Part model, mm, in its own coordinate system. Face numbers are marked on the shaded views. A direction names the side the tool comes from. Coordinates: 2 decimals unless noted, no trailing zeros. Write each loop counter-clockwise with the first axis right and the second up, starting at its lowest first coordinate (ties: lowest second). Pieces come first, ordered by that corner, then holes. Notation, with made-up numbers: M 81.5,67.25 L 92.5,67.25 A10 ccw 92.5,73.25 Z; hole C 82.25,-39 d4. An arc over 180 degrees is marked long. Use a Markdown table: item, result. Add a question column.
Q1. Mould opens along X. For the marked faces 3, 4, 5 and 6 say: released by +X, released by -X, zero draft, split by the parting line, or undercut.
Q2. Pin check, flat tip, straight feed: pin 1 Ø5.5 at (y, z) = (26, 93.5) entering from +X. Stop position of the tip, or through.
Q3. Slice it at A-A on x = 350. Write the cut outline in (y, z), then the cut area to 3 significant figures.
Q4. Tool access for the marked faces 1 and 2: list every direction of +Z, -Z, +X, -X, +Y, -Y with a clear straight run to the whole face (end or side of a thin tool).
Q5. Wall check: L1, parallel to Y at x = 385, z = -39.5; L2, parallel to Z at x = 312, y = 110; L3, parallel to Z at x = 404, y = 32. Give the ranges that are in metal, low to high. Write a range as from..to.
Q6. Slice it at B-B on y = 112.5. Count the separate pieces of the cut face and the enclosed holes in it, then the cut area to 3 significant figures.
from build123d import *

# Parameters (mm, degrees)
SKETCH_1_W      = 740
SKETCH_1_H      = 190
EXTRUDE_1_DEPTH = 100
SKETCH_2_R      = 14.812408038
EXTRUDE_2_DEPTH = 20
SKETCH_3_W      = 180
SKETCH_3_H      = 100
EXTRUDE_3_DEPTH = 100


with BuildPart() as part:
    # 草图1 → 凸台-拉伸1 (new body)
    with BuildSketch(Plane(origin=(0, 0, 0), x_dir=(1, 0, 0), z_dir=(0, 1, 0))):
        Rectangle(SKETCH_1_W, SKETCH_1_H)
    extrude(amount=EXTRUDE_1_DEPTH)

    # 草图2 → 凸台-拉伸2 (add)
    with BuildSketch(Plane(origin=(0, 100, 0), x_dir=(1, 0, 0), z_dir=(0, 1, 0))):
        with Locations(Location((350, -75, 0), (0, 0, 270))):
            Circle(SKETCH_2_R)
        with Locations(Location((300, -75, 0), (0, 0, 270))):
            Circle(SKETCH_2_R)
        with Locations(Location((250, -75, 0), (0, 0, 270))):
            Circle(SKETCH_2_R)
        with Locations(Location((200, -75, 0), (0, 0, 270))):
            Circle(SKETCH_2_R)
        with Locations(Location((150, -75, 0), (0, 0, 270))):
            Circle(SKETCH_2_R)
        with Locations(Location((100, -75, 0), (0, 0, 270))):
            Circle(SKETCH_2_R)
        with Locations(Location((50, -75, 0), (0, 0, 270))):
            Circle(SKETCH_2_R)
        with Locations(Location((0, -75, 0), (0, 0, 270))):
            Circle(SKETCH_2_R)
        with Locations(Location((-50, -75, 0), (0, 0, 270))):
            Circle(SKETCH_2_R)
        with Locations(Location((-100, -75, 0), (0, 0, 270))):
            Circle(SKETCH_2_R)
        with Locations(Location((-150, -75, 0), (0, 0, 270))):
            Circle(SKETCH_2_R)
        with Locations(Location((-200, -75, 0), (0, 0, 270))):
            Circle(SKETCH_2_R)
        with Locations(Location((-250, -75, 0), (0, 0, 270))):
            Circle(SKETCH_2_R)
        with Locations(Location((-300, -75, 0), (0, 0, 270))):
            Circle(SKETCH_2_R)
        with Locations(Location((-350, -75, 0), (0, 0, 270))):
            Circle(SKETCH_2_R)
        with Locations(Location((300, -25, 0), (0, 0, 270))):
            Circle(SKETCH_2_R)
        with Locations(Location((250, -25, 0), (0, 0, 270))):
            Circle(SKETCH_2_R)
        with Locations(Location((200, -25, 0), (0, 0, 270))):
            Circle(SKETCH_2_R)
        with Locations(Location((150, -25, 0), (0, 0, 270))):
            Circle(SKETCH_2_R)
        with Locations(Location((100, -25, 0), (0, 0, 270))):
            Circle(SKETCH_2_R)
        with Locations(Location((50, -25, 0), (0, 0, 270))):
            Circle(SKETCH_2_R)
        with Locations(Location((0, -25, 0), (0, 0, 270))):
            Circle(SKETCH_2_R)
        with Locations(Location((-50, -25, 0), (0, 0, 270))):
            Circle(SKETCH_2_R)
        with Locations(Location((-100, -25, 0), (0, 0, 270))):
            Circle(SKETCH_2_R)
        with Locations(Location((-150, -25, 0), (0, 0, 270))):
            Circle(SKETCH_2_R)
        with Locations(Location((-200, -25, 0), (0, 0, 270))):
            Circle(SKETCH_2_R)
        with Locations(Location((-250, -25, 0), (0, 0, 270))):
            Circle(SKETCH_2_R)
        with Locations(Location((-300, -25, 0), (0, 0, 270))):
            Circle(SKETCH_2_R)
        with Locations(Location((-350, -25, 0), (0, 0, 270))):
            Circle(SKETCH_2_R)
        with Locations(Location((300, 25, 0), (0, 0, 270))):
            Circle(SKETCH_2_R)
        with Locations(Location((250, 25, 0), (0, 0, 270))):
            Circle(SKETCH_2_R)
        with Locations(Location((200, 25, 0), (0, 0, 270))):
            Circle(SKETCH_2_R)
        with Locations(Location((150, 25, 0), (0, 0, 270))):
            Circle(SKETCH_2_R)
        with Locations(Location((100, 25, 0), (0, 0, 270))):
            Circle(SKETCH_2_R)
        with Locations(Location((50, 25, 0), (0, 0, 270))):
            Circle(SKETCH_2_R)
        with Locations(Location((0, 25, 0), (0, 0, 270))):
            Circle(SKETCH_2_R)
        with Locations(Location((-50, 25, 0), (0, 0, 270))):
            Circle(SKETCH_2_R)
        with Locations(Location((-100, 25, 0), (0, 0, 270))):
            Circle(SKETCH_2_R)
        with Locations(Location((-150, 25, 0), (0, 0, 270))):
            Circle(SKETCH_2_R)
        with Locations(Location((-200, 25, 0), (0, 0, 270))):
            Circle(SKETCH_2_R)
        with Locations(Location((-250, 25, 0), (0, 0, 270))):
            Circle(SKETCH_2_R)
        with Locations(Location((-300, 25, 0), (0, 0, 270))):
            Circle(SKETCH_2_R)
        with Locations(Location((-350, 25, 0), (0, 0, 270))):
            Circle(SKETCH_2_R)
        with Locations(Location((300, 75, 0), (0, 0, 270))):
            Circle(SKETCH_2_R)
        with Locations(Location((250, 75, 0), (0, 0, 270))):
            Circle(SKETCH_2_R)
        with Locations(Location((200, 75, 0), (0, 0, 270))):
            Circle(SKETCH_2_R)
        with Locations(Location((150, 75, 0), (0, 0, 270))):
            Circle(SKETCH_2_R)
        with Locations(Location((100, 75, 0), (0, 0, 270))):
            Circle(SKETCH_2_R)
        with Locations(Location((50, 75, 0), (0, 0, 270))):
            Circle(SKETCH_2_R)
        with Locations(Location((0, 75, 0), (0, 0, 270))):
            Circle(SKETCH_2_R)
        with Locations(Location((-50, 75, 0), (0, 0, 270))):
            Circle(SKETCH_2_R)
        with Locations(Location((-100, 75, 0), (0, 0, 270))):
            Circle(SKETCH_2_R)
        with Locations(Location((-150, 75, 0), (0, 0, 270))):
            Circle(SKETCH_2_R)
        with Locations(Location((-200, 75, 0), (0, 0, 270))):
            Circle(SKETCH_2_R)
        with Locations(Location((-250, 75, 0), (0, 0, 270))):
            Circle(SKETCH_2_R)
        with Locations(Location((-300, 75, 0), (0, 0, 270))):
            Circle(SKETCH_2_R)
        with Locations(Location((-350, 75, 0), (0, 0, 270))):
            Circle(SKETCH_2_R)
        with Locations(Location((350, -25, 0), (0, 0, 270))):
            Circle(SKETCH_2_R)
        with Locations(Location((350, 25, 0), (0, 0, 270))):
            Circle(SKETCH_2_R)
        with Locations(Location((350, 75, 0), (0, 0, 270))):
            Circle(SKETCH_2_R)
    extrude(amount=EXTRUDE_2_DEPTH)

    # 草图3 → 凸台-拉伸3 (add)
    with BuildSketch(Plane(origin=(370, 0, 0), x_dir=(0, 0, -1), z_dir=(1, 0, 0))):
        with Locations((0, 50)):
            Rectangle(SKETCH_3_W, SKETCH_3_H)
    extrude(amount=EXTRUDE_3_DEPTH)


solid = part.part
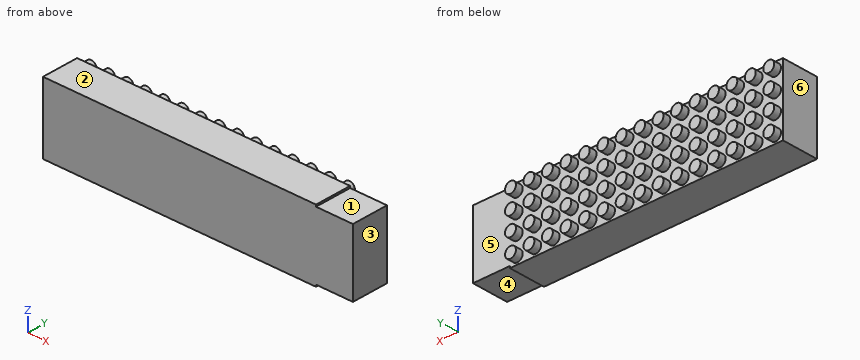
Recorded:
| question | item | result |
|---|---|---|
| 1 | face 3 | released by +X |
| 1 | face 4 | zero draft |
| 1 | face 5 | undercut |
| 1 | face 6 | released by -X |
| 2 | pin 1 | x = 370 |
| 3 | outline | M 0,-95 L 100,-95 L 100,-89.81 L 120,-89.81 L 120,-60.19 L 100,-60.19 L 100,-39.81 L 120,-39.81 L 120,-10.19 L 100,-10.19 L 100,10.19 L 120,10.19 L 120,39.81 L 100,39.81 L 100,60.19 L 120,60.19 L 120,89.81 L 100,89.81 L 100,95 L 0,95 Z |
| 3 | area | 21,400 mm² |
| 4 | face 1 | +Z, +X, +Y, -Y |
| 4 | face 2 | +Z, +X, -X, +Y, -Y |
| 5 | L1 | 0..100 |
| 5 | L2 | -83.68..-66.32, -33.68..-16.32, 16.32..33.68, 66.32..83.68 |
| 5 | L3 | -90..90 |
| 6 | separate pieces | 60 |
| 6 | enclosed holes | 0 |
| 6 | area | 41,400 mm² |
